```python
from build123d import *

# Parameters (mm, degrees)
RESSALTO_EXTRUS_O1_REACH      = 37.374
RESSALTO_EXTRUS_O1_END_RADIUS = 13.453624047
ESBO_O2_R                     = 3.175
CHANFRO1_SIZE                 = 0.5


with BuildPart() as part:
    # Esboço1 → Revolução1 (revolve)
    with BuildSketch(Plane.XY, mode=Mode.PRIVATE) as revolu_o1_sk:
        with BuildLine():
            Line((-9, 10), (-9, 8))
            Line((-9, 8), (9, 8))
            Line((9, 8), (9, 10))
            ThreePointArc((9, 10), (0, 13.453624047), (-9, 10))
        make_face()
    revolve(revolu_o1_sk.sketch.rotate(Axis((0, 0, 0), (1, 0, 0)), 90), axis=Axis((0, 0, 0), (1, 0, 0)))

    # Ressalto-extrusão1: up to this sphere (the profile starts outside it)
    ressalto_extrus_o1_end = Location((0, 0, 0)) * Sphere(RESSALTO_EXTRUS_O1_END_RADIUS, mode=Mode.PRIVATE)
    # Esboço2 → Ressalto-extrusão1 (add, up to the surface)
    with BuildSketch(Plane(origin=(0, 18, 0), x_dir=(1, 0, 0), z_dir=(0, 1, 0)), mode=Mode.PRIVATE) as ressalto_extrus_o1_sk1:
        with Locations(Location((0, 0, 0), (0, 0, 270))):
            Circle(ESBO_O2_R)
    ressalto_extrus_o1_tool1 = extrude(ressalto_extrus_o1_sk1.sketch, amount=-RESSALTO_EXTRUS_O1_REACH, mode=Mode.PRIVATE) - ressalto_extrus_o1_end
    add(ressalto_extrus_o1_tool1.solids().sort_by_distance((0, 18, 0))[0])

    # Chanfro1
    chanfro1_edges = [part.edges().sort_by_distance(p)[0] for p in [
        (0, 18, -3.175),
    ]]
    chamfer(chanfro1_edges, length=CHANFRO1_SIZE)


solid = part.part
```
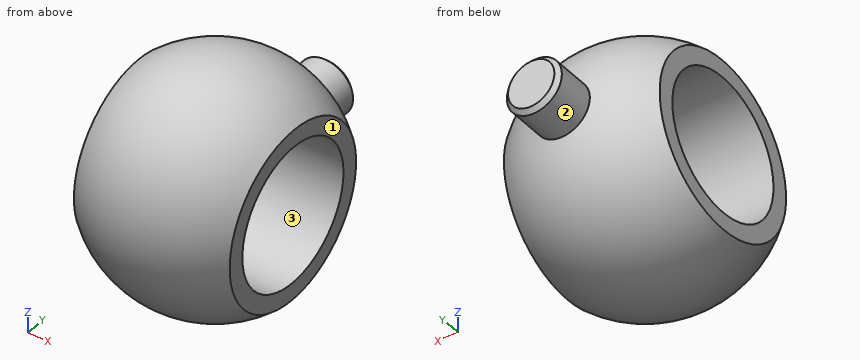
CAD build for the part. Positions are in the model's coordinates, mm. Face numbers are marked on the shaded views. Coordinates: 2 decimals unless noted, no trailing zeros. Loops run counter-clockwise (first coordinate to the right, second up) from the corner with the lowest first, then second, coordinate; pieces in that order, holes last. Notation, with made-up numbers: (-27.5, 25.5) - (-14.5, 25.5) arc R33 cw to (-14.5, 62.5) - close; hole circle Ø5 at (36, 8.5). An arc over 180 degrees is marked (long way). Return JSON: item names as keys, results as strings.
1. Band-saw the part on C-C (y = 0). Give the cut face in (x, z), and give its area (3 significant figures).
Result:
{"outline": "(-9, -10) arc R13.45 ccw to (9, -10) - (9, -8) - (-9, -8) - close; (-9, 8) - (9, 8) - (9, 10) arc R13.45 ccw to (-9, 10) - close", "area": "157 mm2"}
2. Band-saw the part on D-D (z = -7). Give the cut face in (x, y).
Result:
{"outline": "(-9, -7.14) arc R11.49 ccw to (9, -7.14) - (9, -3.87) - (-9, -3.87) - close; (-9, 3.87) - (9, 3.87) - (9, 7.14) arc R11.49 ccw to (-9, 7.14) - close"}
3. Probe L1, parallel to Y at x = 3, z = 0 (3 decimals); L2, parallel to Z at x = -0.75, y = 4; L3, parallel to Y at x = -1.75, z = -2. List the from-to ranges inside material, lowest first. Write a range as from..to.
Result:
{"L1": "y = -13.115..-8, 8..17.675", "L2": "z = -12.82..-6.93, 6.93..12.82", "L3": "y = -13.19..-7.75, 7.75..18"}
4. Drop flat-ended pins along their axis: pin 1 (1.5 mm diameter, centred on x = 0, y = 12.5, fed in from -Z); pin 2 (2 mm diameter, centred on y = -4.5, z = -6, fed in from +X); pin 3 (8 mm diameter, centred on x = -5, y = 12, fed in from +Z); pin 4 (13 mm diameter, centred on y = 0, z = 0, fed in from -X). Give the stop position or say it passes through.
Result:
{"pin 1": "stops at z = -6.55", "pin 2": "stops at x = 9", "pin 3": "stops at z = 10", "pin 4": "passes through"}
5. Mould opens along Z. For the marked faces 1, 2 and 3 say: released by +Z, released by -Z, zero draft, split by the parting line, or undercut.
Result:
{"face 1": "zero draft", "face 2": "split by the parting line", "face 3": "undercut"}
6. Band-saw the part on B-B (z = 0). Give the cut face in (x, y) (3 decimals), and give its area (3 significant figures).
Result:
{"outline": "(-9, -10) arc R13.454 ccw to (9, -10) - (9, -8) - (-9, -8) - close; (-9, 8) - (9, 8) - (9, 10) arc R13.454 ccw to (3.175, 13.074) - (3.175, 17.5) - (2.675, 18) - (-2.675, 18) - (-3.175, 17.5) - (-3.175, 13.074) arc R13.454 ccw to (-9, 10) - close", "area": "187 mm2"}
7. Band-saw the part on A-A (x = 0). Give the cut face in (y, z) (3 decimals), and give its area (3 significant figures).
Result:
{"outline": "(13.074, -3.175) - (17.5, -3.175) - (18, -2.675) - (18, 2.675) - (17.5, 3.175) - (13.074, 3.175) arc R13.454 ccw (long way) to start; hole circle Ø16 at (0, 0)", "area": "397 mm2"}
